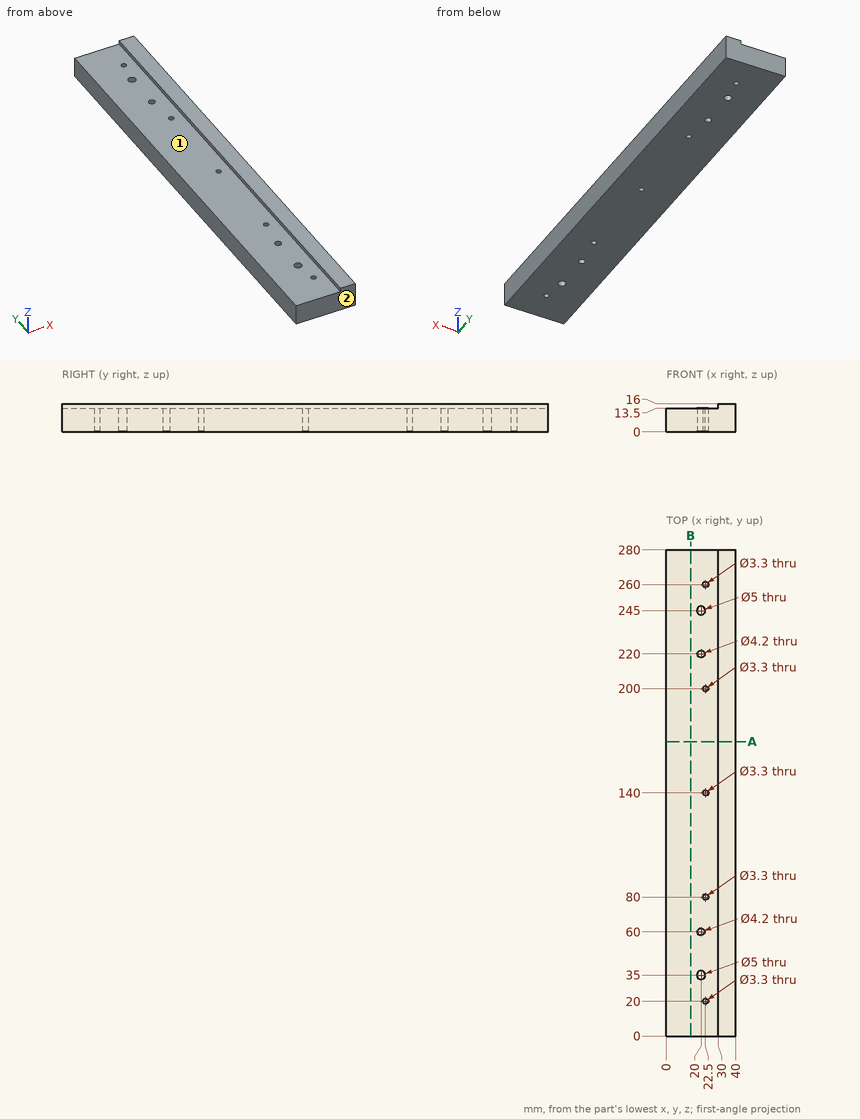
Geometry check sheet. Reference: drawing and pictorial views, mm from the part's lowest x, y, z. A direction names the side the tool comes from. Round coordinates to 2 decimals unless told otherwise and drop trailing zeros. Loops run counter-clockwise (first coordinate to the right, second up) from the corner with the lowest first, then second, coordinate; pieces in that order, holes last. Notation, with made-up numbers: M -17.75,49.5 L 4.25,49.5 A16 cw 4.25,55.5 Z; hole C 51.5,88.25 d10. An arc over 180 degrees is marked long. One line per item, written item: value.
(1) Depth check by flat-ended pin: pin 1 Ø0.8 at (y, z) = (202, 15) entering from -X; pin 2 Ø15 at (x, y) = (15.5, 177) entering from +Z. Enter the tip coordinate at first touch or a pass-through.
Computed values:
pin 1: stops at x = 30
pin 2: stops at z = 13.5
(2) Sectioned sample at B-B, the plane x = 14. Record the cut outline in (y, z), then the cut area to 3 significant figures.
Computed values:
outline: M 0,0 L 280,0 L 280,13.5 L 0,13.5 Z
area: 3,780 mm^2
(3) Access from +Z, -Z, +X, -X, +Y, -Y to the whole of each face (thin tool, end or side, straight path). Record for the marked faces 1 and 2.
Computed values:
face 1: +Z, -X, +Y, -Y
face 2: +Z, -Z, +X, -X, -Y
(4) Thickness scan on line 1 (Y direction, x = 20, z = 8.5); line 2 (X direction, y = 220, z = 10); line 3 (X direction, y = 80, z = 9.25). Record the ranges inside material, lowest first.
Computed values:
line 1: y = 0 to 32.5, 37.5 to 57.9, 62.1 to 217.9, 222.1 to 242.5, 247.5 to 280
line 2: x = 0 to 17.9, 22.1 to 40
line 3: x = 0 to 20.85, 24.15 to 40
(5) Sectioned sample at A-A, the plane y = 169.5. Record the cut outline in (x, z), then the cut area to 3 significant figures.
Computed values:
outline: M 0,0 L 40,0 L 40,16 L 30,16 L 30,13.5 L 0,13.5 Z
area: 565 mm^2
